```python
from build123d import *

# Parameters (mm, degrees)
F0_W     = 140
F0_H     = 63
F1_DEPTH = 1.75
F2_W     = 140
F2_H     = 63
F2_W_2   = 136.5
F2_H_2   = 59.5
F3_DEPTH = 25
F4_R     = 0.7
F5_SIZE  = 2


with BuildPart() as f1:
    # F0 (on Top) → F1 (new body)
    with BuildSketch(Plane.XY):
        with Locations((2.7499999851, -32.9423031422)):
            Rectangle(F0_W, F0_H)
    extrude(amount=F1_DEPTH)

    # F2 (on face) → F3 (join)
    with BuildSketch(Plane.XY.offset(1.75)):
        with Locations((2.7499999851, -32.9423031422)):
            Rectangle(F2_W, F2_H)
        with Locations((2.7499999851, -32.9423031422)):
            Rectangle(F2_W_2, F2_H_2, mode=Mode.SUBTRACT)
    extrude(amount=F3_DEPTH)

    # F4
    f4_edges = [f1.edges().sort_by_distance(p)[0] for p in [
        (2.75, -1.442303, 26.75),
        (72.75, -32.942303, 26.75),
        (2.75, -64.442303, 26.75),
        (-67.25, -32.942303, 26.75),
    ]]
    fillet(f4_edges, radius=F4_R)

    # F5
    f5_edges = [f1.edges().sort_by_distance(p)[0] for p in [
        (2.75, -1.442303, 0),
        (-67.25, -32.942303, 0),
        (2.75, -64.442303, 0),
        (72.75, -32.942303, 0),
    ]]
    chamfer(f5_edges, length=F5_SIZE)


solid = f1.part
```
Geometry check sheet. Reference: the model listing, model coordinates, mm. A direction names the side the tool comes from. Give positions to 0.01 mm unless a question says otherwise; leave off trailing zeros. Order: outer loops, then holes, each group sorted by start corner. A loop starts at its lowest first (then second) coordinate and runs counter-clockwise, first axis right, second up. Notation, with made-up numbers: (46.25, 45.25) - (63.25, 45.25) arc R23 ccw to (63.25, 75.25) - close; hole circle Ø3 at (17.25, 78). An arc over 180 degrees is marked (long way). Answer in a Markdown table with one row per item. Add a question column.
Q1. Cross-section at C-C, the plane x = 36. Enter the section's corners in (y, z).
Q2. Tool access check on faces 4 (the flat face through (2, -3, 26.75)), 5 (the flat face through (-65.5, -33, 14)). Record the directions out of +Z, -Z, +X, -X, +Y, -Y that give a thin tool (end or side, any length) a straight path to the whole face; none if there is none.
Q3. Cross-section at B-B, the plane y = -27.5. Enter the section's corners in (x, z), then the cut area to 3 significant figures.
Q4. Cross-section at A-A, the plane z = 18. Enter the section's corners in (x, y).
Q5. Material ranges on probe 1 along X at (y, z) = (-22.5, 17); probe 2 along Y at (x, z) = (14, 24.25); probe 3 along Z at (x, y) = (7, -44), recorded low to high. Write a range as from..to.
Q6. Mould release check, pull along Y, two halves, no side actions. Record for faces 1 (the flat face through (71, -33, 14)), 2 (the flat face through (-67.25, -33, 14)), 3 (the flat face through (2, -1.442, 14)): pulls with the +Y half, pulls with the -Y half, needs draft (parallel to the pull), parting line crosses it, or undercut.
Check values:
| question | item | result |
|---|---|---|
| 1 | outline | (-64.44, 2) - (-62.44, 0) - (-3.44, 0) - (-1.44, 2) - (-1.44, 26.05) arc R0.7 ccw to (-2.14, 26.75) - (-3.19, 26.75) - (-3.19, 1.75) - (-62.69, 1.75) - (-62.69, 26.75) - (-63.74, 26.75) arc R0.7 ccw to (-64.44, 26.05) - close |
| 2 | face 4 | +Z, +X, -X, +Y, -Y |
| 2 | face 5 | +Z |
| 3 | outline | (-67.25, 2) - (-65.25, 0) - (70.75, 0) - (72.75, 2) - (72.75, 26.05) arc R0.7 ccw to (72.05, 26.75) - (71, 26.75) - (71, 1.75) - (-65.5, 1.75) - (-65.5, 26.75) - (-66.55, 26.75) arc R0.7 ccw to (-67.25, 26.05) - close |
| 3 | area | 328 mm^2 |
| 4 | outline | (-67.25, -64.44) - (72.75, -64.44) - (72.75, -1.44) - (-67.25, -1.44) - close; hole (-65.5, -62.69) - (71, -62.69) - (71, -3.19) - (-65.5, -3.19) - close |
| 5 | probe 1 | x = -67.25..-65.5, 71..72.75 |
| 5 | probe 2 | y = -64.44..-62.69, -3.19..-1.44 |
| 5 | probe 3 | z = 0..1.75 |
| 6 | face 1 | undercut |
| 6 | face 2 | needs draft |
| 6 | face 3 | pulls with the +Y half |
